The model under review builds one solid part; all positions refer to its coordinate system, in mm. A direction names the side the tool comes from. Round coordinates to 2 decimals unless told otherwise and drop trailing zeros. Write each loop counter-clockwise with the first axis right and the second up, starting at its lowest first coordinate (ties: lowest second). Pieces come first, ordered by that corner, then holes. Notation, with made-up numbers: (55, 67) -> (108, 67) arc R19 cw to (108, 85) -> close; hole circle Ø10 at (76, 82.25). An arc over 180 degrees is marked (long way). Answer in a Markdown table with one row per item. Add a question column.
```python
from build123d import *

# Parameters (mm, degrees)
ESBO_O1_R                = 80
ESBO_O1_R_2              = 50
RESSALTO_EXTRUS_O1_DEPTH = 50
FILETE1_R                = 15
CASCA1_T                 = 3


with BuildPart() as part:
    # Esboço1 → Ressalto-extrusão1 (new body)
    with BuildSketch(Plane(origin=(0, 0, 0), x_dir=(0, 0, -1), z_dir=(1, 0, 0))):
        Circle(ESBO_O1_R)
        Circle(ESBO_O1_R_2, mode=Mode.SUBTRACT)
    extrude(amount=RESSALTO_EXTRUS_O1_DEPTH)

    # Filete1
    filete1_edges = [part.edges().sort_by_distance(p)[0] for p in [
        (50, 0, 80),
        (0, 0, 80),
    ]]
    fillet(filete1_edges, radius=FILETE1_R)

    # Casca1 (no face opened: a closed hollow body)
    add(offset(amount=-CASCA1_T, mode=Mode.PRIVATE), mode=Mode.SUBTRACT)


solid = part.part
```
1. Insertion check: pin 1 Ø2 at (x, y) = (30, 6.5) entering from +Z; pin 2 Ø4 at (x, y) = (22, 2.5) entering from -Z; pin 3 Ø5 at (x, z) = (13.5, -57.5) entering from -Y. Each pin has a flat end and moves straight along its axis. Give the tip position at first contact, or say it passes through.
2. Add section C-C on x = 29. Write out the cut boundary in (y, z), plus the area to 3 significant figures.
3. Mouldability with a two-part tool opening along X and no side actions: class faces 3 (the cylindrical face through (24.86, -78.1, 17.34)), 4 (the flat face through (0, -38, -33)), 5 (the cylindrical face through (24.86, -46.853, 61.105)) as pulls with the +X half, pulls with the -X half, needs draft (parallel to the pull), parting line crosses it, or undercut.
4. Add section D-D on x = 12. Write out the cut boundary in (y, z).
5. Add section A-A on y = 0. Write out the cut boundary in (x, z).
6. Tool access review of faces 1 (the cylindrical face through (24.65, 15.02, -47.69)), 2 (the cylindrical face through (25, 45, -28)): name each direction out of +Z, -Z, +X, -X, +Y, -Y from which nothing blocks a thin tool from reaching the whole face with its end or side.
7. For L1, parallel to Y at x = 27, z = 0; L2, parallel to X at y = 65, z = -10.5; L3, parallel to Z at x = 22.5, y = -16, list the stretches that pass through material, from the lowest coordinate up.
Filled in:
| question | item | result |
|---|---|---|
| 1 | pin 1 | z = 79.81 |
| 1 | pin 2 | z = -80 |
| 1 | pin 3 | y = -58.01 |
| 2 | outline | circle Ø160 at (0, 0); circle Ø106 at (0, 0); hole circle Ø154 at (0, 0); hole circle Ø100 at (0, 0) |
| 2 | area | 2,450 mm² |
| 3 | face 3 | needs draft |
| 3 | face 4 | pulls with the -X half |
| 3 | face 5 | undercut |
| 4 | outline | circle Ø159.39 at (0, 0); circle Ø106 at (0, 0); hole circle Ø153.24 at (0, 0); hole circle Ø100 at (0, 0) |
| 5 | outline | (0, -65) arc R15 ccw to (15, -80) -> (35, -80) arc R15 ccw to (50, -65) -> (50, -50) -> (0, -50) -> close; (0, 50) -> (50, 50) -> (50, 65) arc R15 ccw to (35, 80) -> (15, 80) arc R15 ccw to (0, 65) -> close; hole (3, -65) arc R12 ccw to (15, -77) -> (35, -77) arc R12 ccw to (47, -65) -> (47, -53) -> (3, -53) -> close; hole (3, 53) -> (47, 53) -> (47, 65) arc R12 ccw to (35, 77) -> (15, 77) arc R12 ccw to (3, 65) -> close |
| 6 | face 1 | +X, -X |
| 6 | face 2 | none |
| 7 | L1 | -80 to -77, -53 to -50, 50 to 53, 77 to 80 |
| 7 | L2 | 0.02 to 3.03, 46.97 to 49.98 |
| 7 | L3 | -78.38 to -75.32, -50.53 to -47.37, 47.37 to 50.53, 75.32 to 78.38 |
